Source: CAD feature listing. Evaluate the final solid. Frame: model axes, mm. Round coordinates to 2 decimals unless told otherwise and drop trailing zeros. Write each loop counter-clockwise with the first axis right and the second up, starting at its lowest first coordinate (ties: lowest second). Pieces come first, ordered by that corner, then holes. Notation, with made-up numbers: (27, -30.5) -> (45, -30.5) arc R23 ccw to (45, 4.5) -> close; hole circle Ø1 at (46, 63.5). An arc over 180 degrees is marked (long way). Put each result on its own line as item: value.
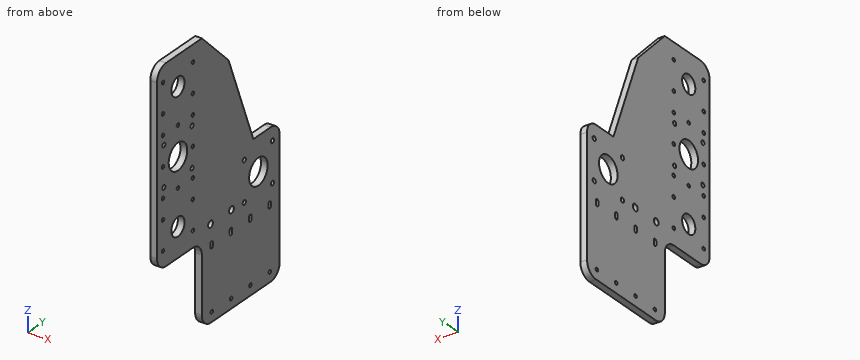
```python
from build123d import *

# Parameters (mm, degrees)
F0_R     = 2.1
F0_R_2   = 11
F0_R_3   = 4
F0_R_4   = 2.65
F0_R_5   = 15.5
F0_R_6   = 2.6
F1_DEPTH = 8


with BuildPart() as f1:
    # F0 (on Right) → F1 (new body)
    with BuildSketch(Plane.YZ):
        with BuildLine():
            ThreePointArc((0, -5), (4.393398, -15.606602), (15, -20))
            Line((15, -20), (115, -20))
            ThreePointArc((115, -20), (125.606602, -15.606602), (130, -5))
            Line((130, -5), (130, 136.83))
            ThreePointArc((130, 136.83), (125.606602, 147.436602), (115, 151.83))
            Line((115, 151.83), (85.92, 151.83))
            Line((85.92, 151.83), (44.487871, 258.512129))
            Line((44.487871, 258.512129), (0, 303))
            Line((0, 303), (-60, 303))
            ThreePointArc((-60, 303), (-70.606602, 298.606602), (-75, 288))
            Line((-75, 288), (-75, 92))
            ThreePointArc((-75, 92), (-70.606602, 81.393398), (-60, 77))
            Line((-60, 77), (-15, 77))
            ThreePointArc((-15, 77), (-4.393398, 72.606602), (0, 62))
            Line((0, 62), (0, -5))
        make_face()
        with Locations((16.54, -8.5)):
            Circle(F0_R, mode=Mode.SUBTRACT)
        with Locations((-65, 96.141)):
            Circle(F0_R, mode=Mode.SUBTRACT)
        with Locations((-65, 130.8)):
            Circle(F0_R, mode=Mode.SUBTRACT)
        with Locations((-40, 111.83)):
            Circle(F0_R_2, mode=Mode.SUBTRACT)
        with Locations((-15, 96.141)):
            Circle(F0_R, mode=Mode.SUBTRACT)
        with BuildLine():
            Line((14.19, 64.078), (14.19, 68.078))
            ThreePointArc((14.19, 68.078), (16.29, 70.178), (18.39, 68.078))
            Line((18.39, 68.078), (18.39, 64.078))
            ThreePointArc((18.39, 64.078), (16.29, 61.978), (14.19, 64.078))
        make_face(mode=Mode.SUBTRACT)
        with Locations((14.43, 89.83)):
            Circle(F0_R_3, mode=Mode.SUBTRACT)
        with Locations((-15, 130.8)):
            Circle(F0_R, mode=Mode.SUBTRACT)
        with Locations((48.86, -8.5)):
            Circle(F0_R, mode=Mode.SUBTRACT)
        with Locations((81.18, -8.5)):
            Circle(F0_R, mode=Mode.SUBTRACT)
        with Locations((113.5, -8.5)):
            Circle(F0_R, mode=Mode.SUBTRACT)
        with BuildLine():
            Line((46.51, 64.078), (46.51, 68.078))
            ThreePointArc((46.51, 68.078), (48.61, 70.178), (50.71, 68.078))
            Line((50.71, 68.078), (50.71, 64.078))
            ThreePointArc((50.71, 64.078), (48.61, 61.978), (46.51, 64.078))
        make_face(mode=Mode.SUBTRACT)
        with Locations((49.43, 89.83)):
            Circle(F0_R_3, mode=Mode.SUBTRACT)
        with Locations((70.86, 88.26)):
            Circle(F0_R_4, mode=Mode.SUBTRACT)
        with Locations((70.86, 135.4)):
            Circle(F0_R_4, mode=Mode.SUBTRACT)
        with BuildLine():
            Line((78.83, 64.078), (78.83, 68.078))
            ThreePointArc((78.83, 68.078), (80.93, 70.178), (83.03, 68.078))
            Line((83.03, 68.078), (83.03, 64.078))
            ThreePointArc((83.03, 64.078), (80.93, 61.978), (78.83, 64.078))
        make_face(mode=Mode.SUBTRACT)
        with BuildLine():
            Line((111.15, 64.078), (111.15, 68.078))
            ThreePointArc((111.15, 68.078), (113.25, 70.178), (115.35, 68.078))
            Line((115.35, 68.078), (115.35, 64.078))
            ThreePointArc((115.35, 64.078), (113.25, 61.978), (111.15, 64.078))
        make_face(mode=Mode.SUBTRACT)
        with Locations((118, 88.26)):
            Circle(F0_R_4, mode=Mode.SUBTRACT)
        with Locations((94.43, 111.83)):
            Circle(F0_R_5, mode=Mode.SUBTRACT)
        with Locations((118, 135.4)):
            Circle(F0_R_4, mode=Mode.SUBTRACT)
        with Locations((-65, 154.72)):
            Circle(F0_R, mode=Mode.SUBTRACT)
        with Locations((-63.57, 166.15)):
            Circle(F0_R_6, mode=Mode.SUBTRACT)
        with Locations((-40, 154.72)):
            Circle(F0_R, mode=Mode.SUBTRACT)
        with Locations((-65, 189.72)):
            Circle(F0_R, mode=Mode.SUBTRACT)
        with Locations((-63.57, 213.29)):
            Circle(F0_R_6, mode=Mode.SUBTRACT)
        with Locations((-40, 189.72)):
            Circle(F0_R_5, mode=Mode.SUBTRACT)
        with Locations((-15, 154.72)):
            Circle(F0_R, mode=Mode.SUBTRACT)
        with Locations((-16.43, 166.15)):
            Circle(F0_R_6, mode=Mode.SUBTRACT)
        with Locations((-15, 189.72)):
            Circle(F0_R, mode=Mode.SUBTRACT)
        with Locations((-16.43, 213.29)):
            Circle(F0_R_6, mode=Mode.SUBTRACT)
        with Locations((-65, 224.72)):
            Circle(F0_R, mode=Mode.SUBTRACT)
        with Locations((-65, 248.64)):
            Circle(F0_R, mode=Mode.SUBTRACT)
        with Locations((-40, 224.72)):
            Circle(F0_R, mode=Mode.SUBTRACT)
        with Locations((-65, 283.299)):
            Circle(F0_R, mode=Mode.SUBTRACT)
        with Locations((-40, 267.61)):
            Circle(F0_R_2, mode=Mode.SUBTRACT)
        with Locations((-15, 224.72)):
            Circle(F0_R, mode=Mode.SUBTRACT)
        with Locations((-15, 248.64)):
            Circle(F0_R, mode=Mode.SUBTRACT)
        with Locations((-15, 283.299)):
            Circle(F0_R, mode=Mode.SUBTRACT)
    extrude(amount=F1_DEPTH)


solid = f1.part
```
Q1. Material intervals for line 1 (Y direction, x = 7.5, z = 111); line 2 (Y direction, x = 2, z = 92); line 3 (Z direction, x = 2.75, y = -31), sorted ascending. Write a range as [from, to].
Ans:
line 1: y = [-75, -50.97], [-29.03, 78.95], [109.91, 130]
line 2: y = [-75, 11.07], [17.79, 46.07], [52.79, 130]
line 3: z = [77, 105.51], [118.15, 177.1], [202.34, 261.29], [273.93, 303]
Q2. Cut plane B-B on x = 2. Give the number of separate pieces and of enclosed holes in the cut face, and give its area (3 significant figures).
Ans:
separate pieces: 1
enclosed holes: 38
area: 44,100 mm^2
Q3. Cut plane A-A on y = 97. Output: boundary loops of the cut face in (x, z).
Ans:
outline: (0, -20) -> (8, -20) -> (8, 96.54) -> (0, 96.54) -> close; (0, 127.12) -> (8, 127.12) -> (8, 151.83) -> (0, 151.83) -> close
Q4. Cut plane C-C on z = 242.5. Output: boundary loops of the cut face in (x, y).
Ans:
outline: (0, -75) -> (8, -75) -> (8, 50.71) -> (0, 50.71) -> close
Q5. Pin query (flat end, axial travel): pin 1 (3 mm diameter, centred on x = 4.5, z = 67, fed in from -Y); pin 2 (2 mm diameter, centred on x = 5.5, z = 65, fed in from -Y); pin 3 (3 mm diameter, centred on x = 5.5, z = 14, fed in from -Y). Return the tip coordinate at first contact, or that it passes through.
Ans:
pin 1: stops at y = -1.48
pin 2: stops at y = -0.54
pin 3: stops at y = 0
